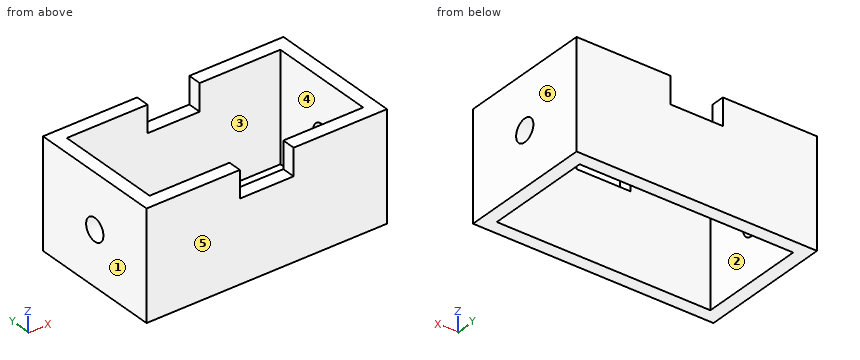
from build123d import *

# Parameters (mm, degrees)
F1_DEPTH = 50.8
F2_W     = 12.7
F2_H     = 12.7
F4_DEPTH = 25.4
F3_W     = 12.7
F3_H     = 12.7
F5_DEPTH = 25.4
F6_R     = 5.295209
F7_DEPTH = 25.4


with BuildPart() as f1:
    # F0 (on Top) → F1 (new body)
    with BuildSketch(Plane.XY):
        Polygon((-50.420101, -10.057684), (-50.420101, 40.742316), (0.379899, 40.742316), (0.379899, 47.092316), (-56.770101, 47.092316), (-56.770101, 15.342316), (-56.770101, -16.407684), (0, -16.407684), (0, -10.057684), align=None)
    extrude(amount=F1_DEPTH)

    # F2 (on face) → F4 (cut)
    with BuildSketch(Plane.XZ.offset(16.407684)):
        with Locations((-6.35, 44.45)):
            Rectangle(F2_W, F2_H)
    extrude(amount=-F4_DEPTH, mode=Mode.SUBTRACT)

    # F3 (on face) → F5 (cut)
    with BuildSketch(Plane(origin=(0, 47.092316, 0), x_dir=(-1, 0, 0), z_dir=(0, 1, 0))):
        with Locations((5.970101, 44.45)):
            Rectangle(F3_W, F3_H)
    extrude(amount=-F5_DEPTH, mode=Mode.SUBTRACT)

    # F6 (on face) → F7 (cut)
    with BuildSketch(Plane(origin=(-56.770101, 0, 0), x_dir=(0, -1, 0), z_dir=(-1, 0, 0))):
        with Locations((-15.342316, 25.4)):
            Circle(F6_R)
    extrude(amount=-F7_DEPTH, mode=Mode.SUBTRACT)

    # F8: F1 across face


with BuildPart() as f1_1:
    add(f1.part)
    add(f1.part.mirror(Plane(origin=(0, -13.232684, 19.05), x_dir=(0, 1, 0), z_dir=(1, 0, 0))))


solid = f1_1.part
Source: CAD feature listing. Evaluate the final solid. Frame: model axes, mm. Face numbers are marked on the shaded views. A direction names the side the tool comes from. Round coordinates to 2 decimals unless told otherwise and drop trailing zeros. Order: outer loops, then holes, each group sorted by start corner. A loop starts at its lowest first (then second) coordinate and runs counter-clockwise, first axis right, second up. Notation, with made-up numbers: (-27.5, -40) - (-5.5, -40) arc R27 cw to (-5.5, -14) - close; hole circle Ø8 at (1, 65). An arc over 180 degrees is marked (long way). Use a Markdown table: item, result. Add a question column.
1. Section query C-C (x = 1). Return the cut outline in (y, z).
2. First-contact query: pin 1 (5 mm diameter, centred on x = 0.5, y = 44, fed in from +Z); pin 2 (10 mm diameter, centred on x = -45, y = 0.5, fed in from -Z). Flat tips, straight axial feed; report the tip coordinate or a pass-through.
3. Section query A-A (z = 44). Return the cut outline in (x, y), then the cut area to 3 significant figures.
4. Section query D-D (z = 33). Return the cut outline in (x, y), then the cut area to 3 significant figures.
5. Section query B-B (y = 36). Return the cut outline in (x, z), then the cut area to 3 significant figures.
6. Mould query, pull axis Y, two halves, no side actions, for the marked faces 3, 4, 5 and 6. Classes: +Y half, -Y half, draft (parallel to the pull), parting line (faces both ways), or undercut.
7. Line query: probe 1 along Y at (x, z) = (-18.5, 47); probe 2 along X at (y, z) = (1.5, 14); probe 3 along Y at (x, z) = (53, 25). Output: solid intervals per line, ascending.
8. Set-up query: the marked faces 1 and 2. Return all of +Z, -Z, +X, -X, +Y, -Y with unobstructed straight access to the full face (end or side cutting, diameter ignored); none if empty.
Derived:
| question | item | result |
|---|---|---|
| 1 | outline | (-16.41, 0) - (-10.06, 0) - (-10.06, 38.1) - (-16.41, 38.1) - close; (40.74, 0) - (47.09, 0) - (47.09, 38.1) - (40.74, 38.1) - close |
| 2 | pin 1 | z = 38.1 |
| 2 | pin 2 | through |
| 3 | outline | (-56.77, -16.41) - (-12.7, -16.41) - (-12.7, -10.06) - (-50.42, -10.06) - (-50.42, 40.74) - (-12.32, 40.74) - (-12.32, 47.09) - (-56.77, 47.09) - close; (12.32, 40.74) - (50.42, 40.74) - (50.42, -10.06) - (12.7, -10.06) - (12.7, -16.41) - (56.77, -16.41) - (56.77, 47.09) - (12.32, 47.09) - close |
| 3 | area | 1,770 mm2 |
| 4 | outline | (-56.77, -16.41) - (56.77, -16.41) - (56.77, 47.09) - (-56.77, 47.09) - close; hole (-50.42, -10.06) - (50.42, -10.06) - (50.42, 40.74) - (-50.42, 40.74) - close |
| 4 | area | 2,090 mm2 |
| 5 | outline | (-56.77, 0) - (-50.42, 0) - (-50.42, 50.8) - (-56.77, 50.8) - close; (50.42, 0) - (56.77, 0) - (56.77, 50.8) - (50.42, 50.8) - close |
| 5 | area | 645 mm2 |
| 6 | face 3 | undercut |
| 6 | face 4 | undercut |
| 6 | face 5 | -Y half |
| 6 | face 6 | draft |
| 7 | probe 1 | -16.41 to -10.06, 40.74 to 47.09 |
| 7 | probe 2 | -56.77 to -50.42, 50.42 to 56.77 |
| 7 | probe 3 | -16.41 to 10.06, 20.62 to 47.09 |
| 8 | face 1 | +Z, -Z, -X, +Y, -Y |
| 8 | face 2 | +Z, -Z |
